```python
from build123d import *

# Parameters (mm, degrees)
SKETCH1_W                 = 95.25
SKETCH1_H                 = 95.25
BOSS_EXTRUDE1_DEPTH       = 57.15
SHELL1_T                  = -3.81
SHELL1_THICKNESS_2_FACE_W = 87.63
SHELL1_THICKNESS_2_FACE_H = 87.63
SHELL1_THICKNESS_2_DEPTH  = 2.54
SKETCH2_R                 = 3.048
BOSS_EXTRUDE2_DEPTH       = 22.86
BOSS_EXTRUDE3_START       = -24.13
SKETCH5_R                 = 3.048
BOSS_EXTRUDE3_DEPTH       = 22.86
SKETCH2_3_W               = 95.25
SKETCH2_3_H               = 1.000000032
CUT_EXTRUDE1_DEPTH        = 129.779816062
SKETCH6_W                 = 28.300000042
SKETCH6_H                 = 28.702
CUT_EXTRUDE2_DEPTH        = 4.318
SKETCH7_W                 = 28.300000042
SKETCH7_H                 = 3.81
CUT_EXTRUDE3_DEPTH        = 3.81
BOSS_EXTRUDE4_DEPTH       = 0.762
FILLET1_R                 = 2.54
BOSS_EXTRUDE7_START       = -47.625
BOSS_EXTRUDE7_DEPTH       = 22.225
SKETCH17_OUTSIDE_W        = 128.934
SKETCH17_OUTSIDE_H        = 95.914
SKETCH17_OUTSIDE_W_2      = 15.24
SKETCH17_OUTSIDE_H_2      = 2.159
CUT_EXTRUDE18_DEPTH       = 2.286


with BuildPart() as part:
    # Sketch1 → Boss-Extrude1 (new body)
    with BuildSketch(Plane(origin=(0, 0, 0), x_dir=(1, 0, 0), z_dir=(0, 1, 0))):
        Rectangle(SKETCH1_W, SKETCH1_H)
    extrude(amount=BOSS_EXTRUDE1_DEPTH)

    # Shell1
    shell1_openings = [part.faces().sort_by_distance(p)[0] for p in [
        (0, 57.15, 0),
    ]]
    offset(amount=SHELL1_T, openings=shell1_openings, kind=Kind.INTERSECTION)

    # Shell1 thickness 2 face (on inner face of the shell) → Shell1 thickness 2 (add)
    with BuildSketch(Plane(origin=(0, 3.81, 0), x_dir=(0, 0, -1), z_dir=(0, -1, 0))):
        Rectangle(SHELL1_THICKNESS_2_FACE_W, SHELL1_THICKNESS_2_FACE_H)
    extrude(amount=-SHELL1_THICKNESS_2_DEPTH)

    # Sketch2 → Boss-Extrude2 (add)
    with BuildSketch(Plane.ZY.offset(47.625)):
        with BuildLine():
            ThreePointArc((-50.165, 57.15), (-57.189031836, 61.843308025), (-58.837102448, 53.557897552))
            Line((-58.837102448, 53.557897552), (-47.625, 42.345795103))
            Line((-47.625, 42.345795103), (-47.625, 56.149999968))
            Line((-47.625, 56.149999968), (-50.264397633, 56.149999968))
            ThreePointArc((-50.264397633, 56.149999968), (-50.189910484, 56.647536083), (-50.165, 57.15))
        make_face()
        with Locations((-55.245, 57.15)):
            Circle(SKETCH2_R, mode=Mode.SUBTRACT)
    extrude(amount=-BOSS_EXTRUDE2_DEPTH)

    # Sketch5 → Boss-Extrude3 (add)
    with BuildSketch(Plane(origin=(47.625, 0, 0), x_dir=(0, 0, -1), z_dir=(1, 0, 0)).offset(BOSS_EXTRUDE3_START)):
        with BuildLine():
            Line((47.625, 56.149999968), (47.625, 42.345795103))
            Line((47.625, 42.345795103), (58.837102448, 53.557897552))
            ThreePointArc((58.837102448, 53.557897552), (56.715282878, 62.012578355), (50.264397633, 56.149999968))
            Line((50.264397633, 56.149999968), (47.625, 56.149999968))
        make_face()
        with Locations(Location((55.245, 57.15, 0), (0, 0, 180))):
            Circle(SKETCH5_R, mode=Mode.SUBTRACT)
    extrude(amount=-BOSS_EXTRUDE3_DEPTH)

    # Sketch2_3 → Cut-Extrude1 (cut, through all)
    with BuildSketch(Plane.ZY.offset(47.625)):
        with Locations((0, 56.649999984)):
            Rectangle(SKETCH2_3_W, SKETCH2_3_H)
    extrude(amount=-CUT_EXTRUDE1_DEPTH, mode=Mode.SUBTRACT)

    # Sketch6 → Cut-Extrude2 (cut)
    with BuildSketch(Plane.XZ):
        with Locations((0, -29.464)):
            Rectangle(SKETCH6_W, SKETCH6_H)
    extrude(amount=-CUT_EXTRUDE2_DEPTH, mode=Mode.SUBTRACT)

    # Sketch7 → Cut-Extrude3 (cut)
    with BuildSketch(Plane(origin=(0, 4.318, 0), x_dir=(-1, 0, 0), z_dir=(0, -1, 0))):
        with Locations((0, 41.91)):
            Rectangle(SKETCH7_W, SKETCH7_H)
    extrude(amount=-CUT_EXTRUDE3_DEPTH, mode=Mode.SUBTRACT)

    # Sketch8 → Boss-Extrude4 (add)
    with BuildSketch(Plane.XZ):
        Polygon((-11.610000021, -15.113), (-14.150000021, -15.113), (-14.150000021, -20.595), (-14.150000021, -28.57736709), (-11.610000021, -28.57736709), (-11.610000021, -20.193), (11.610000021, -20.193), (11.610000021, -28.57736709), (14.150000021, -28.57736709), (14.150000021, -20.595), (14.150000021, -15.113), (11.610000021, -15.113), align=None)
    extrude(amount=-BOSS_EXTRUDE4_DEPTH)

    # Fillet1
    fillet1_edges = [part.edges().sort_by_distance(p)[0] for p in [
        (-47.625, 21.172897552, -47.625),
        (0, 0, -47.625),
        (47.625, 0, 0),
        (0, 0, 47.625),
        (47.625, 28.074999984, -47.625),
        (47.625, 28.074999984, 47.625),
        (-47.625, 28.074999984, 47.625),
        (-47.625, 0, 0),
    ]]
    fillet(fillet1_edges, radius=FILLET1_R)

    # Sketch13 → Boss-Extrude7 (add, symmetric)
    with BuildSketch(Plane.ZY.offset(47.625).offset(BOSS_EXTRUDE7_START)):
        Polygon((47.625, 55.260999968), (47.625, 59.070999968), (49.911, 60.340999968), (49.911, 53.990999968), align=None)
    extrude(amount=BOSS_EXTRUDE7_DEPTH, both=True)

    # Sketch17 outside → Cut-Extrude18 (cut)
    with BuildSketch(Plane.XY.offset(49.911)):
        with Locations((0, 31.115)):
            Rectangle(SKETCH17_OUTSIDE_W, SKETCH17_OUTSIDE_H)
        with Locations((14.605, 55.070499968)):
            Rectangle(SKETCH17_OUTSIDE_W_2, SKETCH17_OUTSIDE_H_2, mode=Mode.SUBTRACT)
    extrude(amount=-CUT_EXTRUDE18_DEPTH, mode=Mode.SUBTRACT)


solid = part.part
```
Input: part model. Units: mm. Frame: model coordinates. A direction names the side the tool comes from. Coordinates: 2 decimals unless noted, no trailing zeros. Write each loop counter-clockwise with the first axis right and the second up, starting at its lowest first coordinate (ties: lowest second). Pieces come first, ordered by that corner, then holes. Notation, with made-up numbers: (48, 89.25) -> (98, 89.25) arc R32 ccw to (98, 118.25) -> close; hole circle Ø4 at (-29, -5.75). An arc over 180 degrees is marked (long way). Answer as a JSON object with one key per item and string values.
1. Section C-C on z = -34.5. Return the cut outline in (x, y) (3 decimals), then the cut area to 3 significant figures.
Result set:
{"outline": "(-47.625, 2.54) arc R2.54 ccw to (-45.085, 0) -> (-14.15, 0) -> (-14.15, 4.318) -> (14.15, 4.318) -> (14.15, 0) -> (45.085, 0) arc R2.54 ccw to (47.625, 2.54) -> (47.625, 56.15) -> (43.815, 56.15) -> (43.815, 6.35) -> (-43.815, 6.35) -> (-43.815, 56.15) -> (-47.625, 56.15) -> close", "area": "859 mm2"}
2. Section B-B on y = 27.5. Return the cut outline in (x, z) (3 decimals), then the cut area to 3 significant figures.
Result set:
{"outline": "(-47.625, -45.085) arc R2.54 ccw to (-45.085, -47.625) -> (45.085, -47.625) arc R2.54 ccw to (47.625, -45.085) -> (47.625, 45.085) arc R2.54 ccw to (45.085, 47.625) -> (-45.085, 47.625) arc R2.54 ccw to (-47.625, 45.085) -> close; hole (-43.815, -43.815) -> (43.815, -43.815) -> (43.815, 43.815) -> (-43.815, 43.815) -> close", "area": "1,390 mm2"}
3. Material intervals for line 1 (X direction, y = 11, z = 42) (3 decimals); line 2 (Z direction, x = -34, y = 57), sorted ascending. Write a range as from..to.
Result set:
{"line 1": "x = -47.625..-43.815, 43.815..47.625", "line 2": "z = -60.32..-58.29, -52.2..-50.17"}
4. Section D-D on x = 41.5. Return the cut outline in (y, z) (3 decimals).
Result set:
{"outline": "(0, -45.085) arc R2.54 ccw to (2.54, -47.625) -> (56.15, -47.625) -> (56.15, -43.815) -> (6.35, -43.815) -> (6.35, 43.815) -> (56.15, 43.815) -> (56.15, 47.625) -> (2.54, 47.625) arc R2.54 ccw to (0, 45.085) -> close"}
5. Section A-A on x = 3.5. Return the cut outline in (y, z) (3 decimals), then the cut area to 3 significant figures.
Result set:
{"outline": "(0, -45.085) arc R2.54 ccw to (2.54, -47.625) -> (42.346, -47.625) -> (53.558, -58.837) arc R5.08 ccw (long way) to (56.15, -50.264) -> (56.15, -43.815) -> (0, -43.815) -> close; (0, -20.193) -> (0.762, -20.193) -> (0.762, -15.113) -> (4.318, -15.113) -> (4.318, -40.005) -> (6.35, -40.005) -> (6.35, 43.815) -> (56.15, 43.815) -> (56.15, 47.625) -> (2.54, 47.625) arc R2.54 ccw to (0, 45.085) -> close; hole circle Ø6.096 at (57.15, -55.245)", "area": "969 mm2"}
6. Mould query, pull axis Z, two halves, no side actions, for faces 4 (the face through (12.225, 61.968, -56.855)), 5 (the face through (-1, 31, 43.815)), 6 (the face through (-47.625, 32, -7)), 7 (the face through (-36.36, 55.98, -52.43)). Classes: released by +Z, released by -Z, zero draft, split by the parting line, or undercut.
Result set:
{"face 4": "split by the parting line", "face 5": "undercut", "face 6": "zero draft", "face 7": "undercut"}
7. Access query for faces 1 (the face through (23.495, 52, -52)), 2 (the face through (0, 3, -15.113)), 3 (the face through (-1, 28, -43.815)). Directions: +Z, -Z, +X, -X, +Y, -Y. A direction counts if a zero-diameter tool reaches every point of the face in a straight line with its end or side. Return the directions, or none.
Result set:
{"face 1": "-Z, +X, +Y, -Y", "face 2": "none", "face 3": "+Y"}
8. First-contact query: P1, Ø0.6, axis at y = 0, z = -25, coming from the +X side; P2, Ø0.6, axis at x = 6.5, y = 5.5, coming from the -Z side (3 decimals); P3, Ø16, axis at x = -19.5, y = 32.5, coming from the +Z side (3 decimals). Flat tips, straight axial feed; report the tip coordinate or a pass-through.
Result set:
{"P1": "stops at x = 46.28", "P2": "stops at z = -47.625", "P3": "stops at z = 47.625"}
